Here's how the part is built. I have some questions about the finished solid (model axes, mm). Round coordinates to 2 decimals unless told otherwise and drop trailing zeros. Write each loop counter-clockwise with the first axis right and the second up, starting at its lowest first coordinate (ties: lowest second). Pieces come first, ordered by that corner, then holes. Notation, with made-up numbers: (-31.75, 50) -> (17.25, 50) arc R5 ccw to (17.25, 54) -> close; hole circle Ø2 at (30.5, -10). An arc over 180 degrees is marked (long way). Put each result on its own line as item: value. Start each with the question number.
1) If I drill on line 1 along X through (y, z) = (1.65, -16); line 2 along Z through (x, y) = (-30, 3.3); line 3 along Z through (x, y) = (-37, 2.85), over which ranges is the centre line in solid material (lowest first)? Write a range as [from, to].
2) Will these pins go through, and if not, where does the flat tip stop? P1, Ø3, axis at x = 30.47, z = -17.5, coming from the -Y side; P2, Ø1, axis at x = 37, y = 4.5, coming from the +Z side; P3, Ø1.2, axis at x = -48.5, y = 1.5, coming from the +Z side; P4, Ø1.2, axis at x = -48.5, y = 2.5, coming from the -Z side.
3) I want a section at B-B, the plane y = 1.2. Give the number of separate pieces and of enclosed holes in the cut face, then the cut area to 3 significant figures.
4) I want a section at A-A, the plane x = 20. List the corners of the cut face in (y, z) for me, then the cut area to 3 significant figures.
from build123d import *

# Parameters (mm, degrees)
F0_R     = 2
F0_R_2   = 12.5
F1_DEPTH = 5
F2_R     = 2


# Not quite as in the source:
# - two fillets or chamfers of one size are made in one step
# - ends of sketch curves that miss each other by under 0.0002 mm in the source are joined


with BuildPart() as f1:
    # F0 (on Front) → F1 (new body)
    with BuildSketch(Plane.XZ):
        with BuildLine():
            Line((30.4688991789, 25), (-33.5311008211, 25))
            ThreePointArc((-33.5311008211, 25), (-58.5311008211, 0), (-33.5311008211, -25))
            Line((-33.5311008211, -25), (30.4688991789, -25))
            ThreePointArc((30.4688991789, -25), (55.4688991789, 0), (30.4688991789, 25))
        make_face()
        with BuildLine():
            ThreePointArc((-31.5311008211, -13), (-29.5311008211, -15), (-31.5311008211, -17))
            Line((-31.5311008211, -17), (-35.5311008211, -17))
            ThreePointArc((-35.5311008211, -17), (-37.5311008211, -15), (-35.5311008211, -13))
            Line((-35.5311008211, -13), (-31.5311008211, -13))
        make_face(mode=Mode.SUBTRACT)
        with BuildLine():
            ThreePointArc((-35.6998849753, 5.0009525442), (-35.5197441178, 5.0037871123), (-35.3396179829, 5.0001348744))
            Line((-35.3396179829, 5.0001348744), (-33.7192871231, 4.9964573365))
            Line((-33.7192871231, 4.9964573365), (-31.8707135701, 4.9922617741))
            ThreePointArc((-31.8707135701, 4.9922617741), (-31.5197441178, 5.0037871123), (-31.1688305974, 4.9906687653))
            ThreePointArc((-31.1688305974, 4.9906687653), (-26.5369680234, -0.310889109), (-31.7905758861, -4.9970678533))
            Line((-31.7905758861, -4.9970678533), (-33.5226571845, -4.9999928705))
            ThreePointArc((-33.5226571845, -4.9999928705), (-33.5268790013, -4.9999982176), (-33.5311008211, -5))
            Line((-33.5311008211, -5), (-35.4576247605, -5.0032605078))
            ThreePointArc((-35.4576247605, -5.0032605078), (-40.5334343372, -0.1211356041), (-35.6998849753, 5.0009525442))
        make_face(mode=Mode.SUBTRACT)
        with Locations((30.4688991789, -17.5)):
            Circle(F0_R, mode=Mode.SUBTRACT)
        with BuildLine():
            ThreePointArc((-46.5311008211, 2), (-44.5311008211, 0), (-46.5311008211, -2))
            Line((-46.5311008211, -2), (-50.5311008211, -2))
            ThreePointArc((-50.5311008211, -2), (-52.5311008211, 0), (-50.5311008211, 2))
            Line((-50.5311008211, 2), (-46.5311008211, 2))
        make_face(mode=Mode.SUBTRACT)
        with BuildLine():
            ThreePointArc((-20.5311008211, -2), (-22.5311008211, 0), (-20.5311008211, 2))
            Line((-20.5311008211, 2), (-16.5311008211, 2))
            ThreePointArc((-16.5311008211, 2), (-14.5311008211, 0), (-16.5311008211, -2))
            Line((-16.5311008211, -2), (-20.5311008211, -2))
        make_face(mode=Mode.SUBTRACT)
        with BuildLine():
            ThreePointArc((-31.5311008211, 17), (-29.5311008211, 15), (-31.5311008211, 13))
            Line((-31.5311008211, 13), (-35.5311008211, 13))
            ThreePointArc((-35.5311008211, 13), (-37.5311008211, 15), (-35.5311008211, 17))
            Line((-35.5311008211, 17), (-31.5311008211, 17))
        make_face(mode=Mode.SUBTRACT)
        with Locations((12.9688991789, 0)):
            Circle(F0_R, mode=Mode.SUBTRACT)
        with Locations((30.4688991789, 0)):
            Circle(F0_R_2, mode=Mode.SUBTRACT)
        with Locations((47.9688991789, 0)):
            Circle(F0_R, mode=Mode.SUBTRACT)
        with Locations((30.4688991789, 17.5)):
            Circle(F0_R, mode=Mode.SUBTRACT)
    extrude(amount=-F1_DEPTH)

    # F2
    f2_edges = [f1.edges().sort_by_distance(p)[0] for p in [
        (55.468899, 5, 0),
        (-1.531101, 0, 25),
        (-1.531101, 5, 25),
        (-58.531101, 5, 0),
        (-1.531101, 5, -25),
        (-1.531101, 0, -25),
        (-58.531101, 0, 0),
        (55.468899, 0, 0),
    ]]
    fillet(f2_edges, radius=F2_R)


solid = f1.part
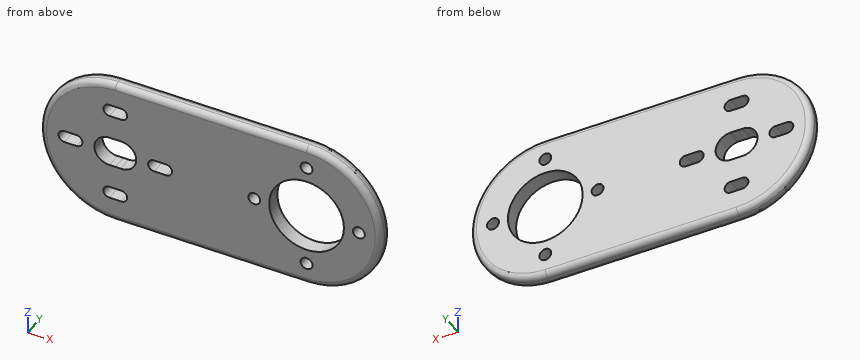
Findings:
1. line 1: x = [-52.7, -37.26], [-29.8, 29.15], [31.79, 49.64]
1. line 2: z = [-24.98, -16.29], [-13.71, -4.76], [4.76, 13.71], [16.29, 24.98]
1. line 3: z = [-24.76, -16.36], [-13.64, -4.78], [4.78, 13.64], [16.36, 24.76]
2. P1: passes through
2. P2: stops at z = 23.88
2. P3: stops at z = 20.41
2. P4: stops at z = -20.46
3. separate pieces: 1
3. enclosed holes: 10
3. area: 4,340 mm2
4. outline: (0, -23) arc R2 ccw to (2, -25) -> (3, -25) arc R2 ccw to (5, -23) -> (5, -6.83) -> (0, -6.83) -> close; (0, 6.83) -> (5, 6.83) -> (5, 23) arc R2 ccw to (3, 25) -> (2, 25) arc R2 ccw to (0, 23) -> close
4. area: 178 mm2
